Could you check a few things on this model? Use its own coordinates, in mm. A direction names the side the tool comes from. Give positions to 0.01 mm unless a question says otherwise; leave off trailing zeros. Loops run counter-clockwise (first coordinate to the right, second up) from the corner with the lowest first, then second, coordinate; pieces in that order, holes last. Notation, with made-up numbers: M 75.5,80 L 130.5,80 A20 ccw 130.5,119 Z; hole C 88,22.25 d2. An arc over 180 degrees is marked long. Use CSV: the item, a comma, the result in double quotes.
```python
from build123d import *

# Parameters (mm, degrees)
ESQUISSE1_W        = 25
ESQUISSE1_H        = 7
BOSS_EXTRU_1_DEPTH = 10
ESQUISSE2_W        = 25
ESQUISSE2_H        = 3
BOSS_EXTRU_2_DEPTH = 1.5


with BuildPart() as part:
    # Esquisse1 → Boss.-Extru.1 (new body)
    with BuildSketch(Plane.XY):
        with Locations((-3.307033874, -4.093457944)):
            Rectangle(ESQUISSE1_W, ESQUISSE1_H)
    extrude(amount=BOSS_EXTRU_1_DEPTH)

    # Esquisse2 → Boss.-Extru.2 (add)
    with BuildSketch(Plane.XZ.offset(7.593457944)):
        with Locations((-3.307033874, 8.5)):
            Rectangle(ESQUISSE2_W, ESQUISSE2_H)
    extrude(amount=BOSS_EXTRU_2_DEPTH)


solid = part.part
```
1. I want a section at A-A, the plane x = 7.25. List the corners of the cut face in (y, z) for me.
Outcome:
outline,"M -9.09,7 L -7.59,7 L -7.59,0 L -0.59,0 L -0.59,10 L -9.09,10 Z"
2. I want a section at C-C, the plane y = -8. List the corners of the cut face in (x, z) for me, then the cut area to 3 significant figures.
Outcome:
outline,"M -15.81,7 L 9.19,7 L 9.19,10 L -15.81,10 Z"
area,"75.0 mm2"
3. I'm going to push flat-ended pins straight in: pin 1 Ø1 at (x, z) = (5.5, 4.5) entering from -Y; pin 2 Ø1.7 at (x, y) = (0, -8.5) entering from -Z. Where does each tip first touch, or does it pass through?
Outcome:
pin 1,"y = -7.59"
pin 2,"z = 7"
4. Please list where these lines run through material, in increasing order: line 1 (Y direction, x = -6, z = 2.25); line 2 (Z direction, x = -0.75, y = -8.25).
Outcome:
line 1,"-7.59 to -0.59"
line 2,"7 to 10"
5. I want a section at B-B, the plane z = 2.25. List the corners of the cut face in (x, y) for me, then the cut area to 3 significant figures.
Outcome:
outline,"M -15.81,-7.59 L 9.19,-7.59 L 9.19,-0.59 L -15.81,-0.59 Z"
area,"175 mm2"
6. Which directions (+Z, -Z, +X, -X, +Y, -Y) give clear straight access to the entire face, cutting with the end or side of a thin tool? Please do faces 1 (the face through (-15.807, -4, 5)), 2 (the face through (-3, -8, 7)).
Outcome:
face 1,"+Z, -Z, -X, +Y, -Y"
face 2,"-Z, +X, -X, -Y"
